from build123d import *

# Parameters (mm, degrees)
SKETCH1_R                  = 5
SHAFT_DEPTH                = 45
SKETCH3_R                  = 12.5
DATUM_DEPTH                = 5
WIRE_SUPPORT_ANGLE         = 10
WIRE_SUPPORT_PATTERN_COUNT = 4
SKETCH6_R                  = 2.6
HOLE_DEPTH                 = 11


with BuildPart() as part:
    # Sketch1 → Shaft (new body)
    with BuildSketch(Plane(origin=(0, 0, 0), x_dir=(1, 0, 0), z_dir=(0, 1, 0))):
        with Locations(Location((0, 0, 0), (0, 0, 90))):
            Circle(SKETCH1_R)
    extrude(amount=SHAFT_DEPTH)

    # Sketch3 → Datum (add)
    with BuildSketch(Plane(origin=(0, 0, 0), x_dir=(-1, 0, 0), z_dir=(0, -1, 0))):
        with Locations(Location((0, 0, 0), (0, 0, 90))):
            Circle(SKETCH3_R)
    extrude(amount=-DATUM_DEPTH)

    # Sketch4 → Wire Support (revolve)
    with BuildSketch(Plane(origin=(0, 0, 0), x_dir=(0, 0, -1), z_dir=(1, 0, 0))):
        with BuildLine():
            Line((7.5, 5), (12.5, 5))
            Line((12.5, 5), (12.5, 6.25))
            ThreePointArc((12.5, 6.25), (11.75, 7), (12.5, 7.75))
            Line((12.5, 7.75), (12.5, 9))
            Line((12.5, 9), (7.5, 9))
            Line((7.5, 9), (7.5, 5))
        make_face()
    wire_support = revolve(axis=Axis((0, 45, 0), (0, 1, 0)), revolution_arc=WIRE_SUPPORT_ANGLE)

    # Wire Support Pattern: Wire Support ×4 about axis
    wire_support_pattern_axis = Axis((0, 45, 0), (0, 1, 0))
    for i in range(1, WIRE_SUPPORT_PATTERN_COUNT):
        add(wire_support.rotate(wire_support_pattern_axis, i * 360 / WIRE_SUPPORT_PATTERN_COUNT))

    # Sketch6 → Hole (cut)
    with BuildSketch(Plane.XZ):
        with Locations(Location((0, 0, 0), (0, 0, 270))):
            Circle(SKETCH6_R)
    extrude(amount=-HOLE_DEPTH, mode=Mode.SUBTRACT)


solid = part.part
Here's how the part is built. I have some questions about the finished solid (model axes, mm). A direction names the side the tool comes from. Coordinates: 2 decimals unless noted, no trailing zeros. Write each loop counter-clockwise with the first axis right and the second up, starting at its lowest first coordinate (ties: lowest second). Pieces come first, ordered by that corner, then holes.
Item 1: I want a section at D-D on x = 9.75. Write out the boundary of the cut face in (y, z), and give its area (3 significant figures).
Item 2: Will these pins go through, and if not, where does the flat tip stop? pin 1 (1.7 mm diameter, centred on x = -10.5, z = 1, fed in from +Y); pin 2 (2 mm diameter, centred on y = 7.5, z = 10.5, fed in from -X); pin 3 (12 mm diameter, centred on x = 6, y = 23.5, fed in from -Z).
Item 3: I want a section at B-B on z = -9.75. Write out the boundary of the cut face in (x, y), and give its area (3 significant figures).
Item 4: If we mould it in two halves opening along Z, with no side actions, what happens to faces 1 (the cylindrical face through (12.454, 8.384, -1.074)), 2 (the flat face through (-10, 9, 1)), 3 (the flat face through (0, 11, 0))? For each: +Z half, -Z half, draft (parallel to the pull), parting line (faces both ways), or undercut.
Item 5: If I drill on line 1 (Y direction, x = 3, z = -10.75); line 2 (Z direction, x = -4.5, y = 10); line 3 (Z direction, x = -1, y = 10.5), over which ranges is the centre line in solid material (lowest first)?
Item 6: I want a section at C-C on y = 15. Write out the boundary of the cut face in (x, z).
Item 7: I want a section at A-A on y = 10. Write out the boundary of the cut face in (x, z).
Item 8: On a 3-axis mill with a long thin cutter (end or side, diameter ignored), from which of +Z, -Z, +X, -X, +Y, -Y can I reach the whole of each face in a straight line? I mean faces 4 (the flat face through (-9.81, 7.03, 1.73)), 5 (the cylindrical face through (0.645, 6.972, 7.472)), 6 (the flat face through (0, 7, -10)), 7 (the flat face through (0, 7, 10)). Say none if no direction works.
Findings below:
1. outline: (0, -7.82) - (5, -7.82) - (5, -1.72) - (9, -1.72) - (9, 0) - (5, 0) - (5, 7.82) - (0, 7.82) - close
1. area: 85.1 mm2
2. pin 1: stops at y = 9
2. pin 2: stops at x = 0
2. pin 3: stops at z = -5
3. outline: (-7.82, 0) - (7.82, 0) - (7.82, 5) - (0, 5) - (0, 9) - (-1.72, 9) - (-1.72, 5) - (-7.82, 5) - close
3. area: 85.1 mm2
4. face 1: -Z half
4. face 2: draft
4. face 3: undercut
5. line 1: y = 0 to 5
5. line 2: z = -2.18 to 2.18
5. line 3: z = -4.9 to -2.4, 2.4 to 4.9
6. outline: circle Ø10 at (0, 0)
7. outline: circle Ø10 at (0, 0); hole circle Ø5.2 at (0, 0)
8. face 4: +Z, +Y
8. face 5: -X, +Y
8. face 6: -Z, +X, +Y
8. face 7: +Z, -X, +Y
